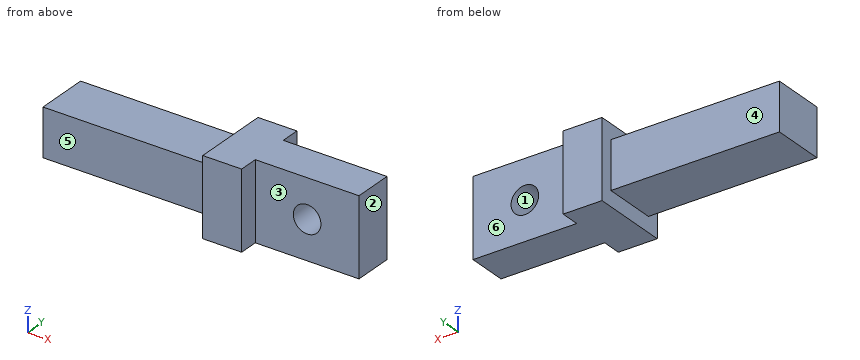
from build123d import *

# Parameters (mm, degrees)
SKETCH1_W               = 19.05
SKETCH1_H               = 19.05
BOSS_EXTRUDE1_DEPTH     = 76.2
SKETCH2_W               = 25.4
SKETCH2_H               = 4.699
CUT_EXTRUDE1_DEPTH      = 81.82230509
SKETCH3_W               = 41.275
SKETCH3_H               = 3.048
CUT_EXTRUDE2_DEPTH      = 81.82230509
SKETCH4_W               = 41.275
SKETCH4_H               = 3.7084
CUT_EXTRUDE3_DEPTH      = 81.158633372
F_1_4_CLEARANCE_HOLE1_D = 6.7564


with BuildPart() as part:
    # Sketch1 → Boss-Extrude1 (new body)
    with BuildSketch(Plane(origin=(0, 0, 0), x_dir=(0, 0, -1), z_dir=(1, 0, 0))):
        with Locations((9.525, 9.525)):
            Rectangle(SKETCH1_W, SKETCH1_H)
    extrude(amount=BOSS_EXTRUDE1_DEPTH)

    # Sketch2 → Cut-Extrude1 (cut, through all)
    with BuildSketch(Plane.XY):
        with Locations((63.5, 16.7005)):
            Rectangle(SKETCH2_W, SKETCH2_H)
        with Locations((63.5, 2.3495)):
            Rectangle(SKETCH2_W, SKETCH2_H)
    extrude(amount=-CUT_EXTRUDE1_DEPTH, mode=Mode.SUBTRACT)

    # Sketch3 → Cut-Extrude2 (cut, through all)
    with BuildSketch(Plane.XY):
        with Locations((20.6375, 17.526)):
            Rectangle(SKETCH3_W, SKETCH3_H)
        with Locations((20.6375, 1.524)):
            Rectangle(SKETCH3_W, SKETCH3_H)
    extrude(amount=-CUT_EXTRUDE2_DEPTH, mode=Mode.SUBTRACT)

    # Sketch4 → Cut-Extrude3 (cut, through all)
    with BuildSketch(Plane(origin=(0, 16.002, 0), x_dir=(1, 0, 0), z_dir=(0, 1, 0))):
        with Locations((20.6375, 17.1958)):
            Rectangle(SKETCH4_W, SKETCH4_H)
        with Locations((20.6375, 1.8542)):
            Rectangle(SKETCH4_W, SKETCH4_H)
    extrude(amount=-CUT_EXTRUDE3_DEPTH, mode=Mode.SUBTRACT)

    # 1/4 Clearance Hole1 (through all)
    with Locations(Plane(origin=(0, 14.351, 0), x_dir=(1, 0, 0), z_dir=(0, 1, 0))):
        with Locations((63.5, 9.525)):
            Hole(F_1_4_CLEARANCE_HOLE1_D / 2)


solid = part.part
Check sheet for the modelled part. Datum: model origin and axes. Units: mm. Face numbers are marked on the shaded views. A direction names the side the tool comes from. Give positions to 0.01 mm unless a question says otherwise; leave off trailing zeros. Loops run counter-clockwise (first coordinate to the right, second up) from the corner with the lowest first, then second, coordinate; pieces in that order, holes last. Notation, with made-up numbers: M 69.25,10 L 75.25,10 A10 ccw 75.25,29 Z; hole C 46,-29.75 d9. An arc over 180 degrees is marked long. Answer as a JSON object with one key per item and string values. Group by question number.
Q1. Cross-section at D-D on y = 3.75. Record the cut outline in (x, z) (3 decimals).
Q2. Go/stop test with flat-tipped pins: P1, Ø1, axis at x = 32.5, z = -6.5, coming from the -Y side; P2, Ø3, axis at x = 13.5, y = 5.5, coming from the -Z side; P3, Ø5.5, axis at x = 63.5, z = -9.525, coming from the +Y side (1 decimal); P4, Ø1.4, axis at y = 3, z = -12, coming from the +X side. Record where each tip stops, or that it passes through.
Q3. Access from +Z, -Z, +X, -X, +Y, -Y to the whole of each face (thin tool, end or side, straight path). Record for the marked faces 4, 5 and 6.
Q4. Material ranges on line 1 along Z through (x, y) = (63.5, 12.75); line 2 along Y through (x, z) = (38, -5); line 3 along Y through (x, z) = (70, -8.75), recorded low to high. Write a range as [from, to].
Q5. Cross-section at A-A on x = 63.5. Record the cut outline in (y, z).
Q6. Release check for a two-part mould opening along X. For the marked faces 1, 2 and 3 record: released by +X, released by -X, zero draft, split by the parting line, or undercut.
Q7. Cross-section at B-B on z = -2. Record the cut outline in (x, y) (3 decimals).
Q8. Cross-section at C-C on y = 8. Record the cut outline in (x, z) (3 decimals).
Evaluation:
{
 "1": {"outline": "M 0,-15.342 L 41.275,-15.342 L 41.275,-19.05 L 50.8,-19.05 L 50.8,0 L 41.275,0 L 41.275,-3.708 L 0,-3.708 Z"},
 "2": {"P1": "stops at y = 3.05", "P2": "stops at z = -15.34", "P3": "passes through", "P4": "stops at x = 50.8"},
 "3": {"face 4": "+Z, -Z, -X, +Y", "face 5": "+Z, -Z, -X, -Y", "face 6": "+Z, -Z, +X, +Y"},
 "4": {"line 1": "z = [-19.05, -12.9], [-6.15, 0]", "line 2": "y = [3.05, 16]", "line 3": "y = [4.7, 14.35]"},
 "5": {"outline": "M 4.7,-19.05 L 14.35,-19.05 L 14.35,-12.9 L 4.7,-12.9 Z; M 4.7,-6.15 L 14.35,-6.15 L 14.35,0 L 4.7,0 Z"},
 "6": {"face 1": "undercut", "face 2": "released by +X", "face 3": "zero draft"},
 "7": {"outline": "M 41.275,0 L 50.8,0 L 50.8,4.699 L 76.2,4.699 L 76.2,14.351 L 50.8,14.351 L 50.8,19.05 L 41.275,19.05 Z"},
 "8": {"outline": "M 0,-15.342 L 41.275,-15.342 L 41.275,-19.05 L 76.2,-19.05 L 76.2,0 L 41.275,0 L 41.275,-3.708 L 0,-3.708 Z; hole C 63.5,-9.525 d6.756"}
}
